```python
from build123d import *

# Parameters (mm, degrees)
FILLET1_R = 0.5


with BuildPart() as part:
    # Sketch1 → Revolve1 (revolve)
    with BuildSketch(Plane.XY):
        Polygon((24.25, 0), (31, 0), (31, 8), (26.75, 8), (26.75, 6), (29.25, 6), (29.25, 4), (26.5, 4), (26.5, 2), (24.25, 2), align=None)
    revolve(axis=Axis((0, 0, 0), (0, 1, 0)))

    # Fillet1
    fillet1_edges = [part.edges().sort_by_distance(p)[0] for p in [
        (-31, 8, 0),
        (-31, 0, 0),
    ]]
    fillet(fillet1_edges, radius=FILLET1_R)


solid = part.part
```
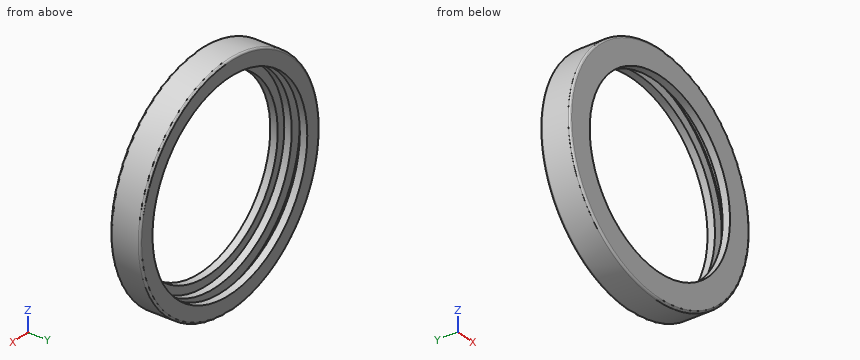
For this review, take the finished solid that the model builds, in its own axes (mm). Give positions to 0.01 mm unless a question says otherwise; leave off trailing zeros. Loops run counter-clockwise (first coordinate to the right, second up) from the corner with the lowest first, then second, coordinate; pieces in that order, holes last. Notation, with made-up numbers: M 10,10.25 L 61,10.25 A12 cw 61,28.25 Z; hole C 18,25.25 d4. An arc over 180 degrees is marked long. One line per item, written item: value. Start each with the question number.
Q1. Clearance check with flat-ended pins moving along their axes: pin 1 Ø1 at (y, z) = (1.5, 15) entering from -X; pin 2 Ø1.5 at (x, y) = (23, 2.5) entering from +Z; pin 3 Ø2 at (y, z) = (2, 15) entering from -X; pin 4 Ø5 at (x, z) = (-12, -17) entering from +Y. State where each tip first meets the part, or that it passes through.
Q2. Add section A-A (x = 0). Give the boundary of the cut face in (y, z).
Q3. Add section B-B (z = 0). Give the boundary of the cut face in (x, y), and give its area (3 significant figures).
Q4. For L1, parallel to Z at x = 0, y = 7.5; L2, parallel to Z at x = 0, y = 4.8, list the stretches that pass through material, from the lowest coordinate up.
Reply:
1. pin 1: x = -27.4
1. pin 2: z = 21.59
1. pin 3: x = -27.66
1. pin 4: through
2. outline: M 0,-30.5 A0.5 ccw 0.5,-31 L 7.5,-31 A0.5 ccw 8,-30.5 L 8,-26.75 L 6,-26.75 L 6,-29.25 L 4,-29.25 L 4,-26.5 L 2,-26.5 L 2,-24.25 L 0,-24.25 Z; M 0,24.25 L 2,24.25 L 2,26.5 L 4,26.5 L 4,29.25 L 6,29.25 L 6,26.75 L 8,26.75 L 8,30.5 A0.5 ccw 7.5,31 L 0.5,31 A0.5 ccw 0,30.5 Z
3. outline: M -31,0.5 A0.5 ccw -30.5,0 L -24.25,0 L -24.25,2 L -26.5,2 L -26.5,4 L -29.25,4 L -29.25,6 L -26.75,6 L -26.75,8 L -30.5,8 A0.5 ccw -31,7.5 Z; M 24.25,0 L 30.5,0 A0.5 ccw 31,0.5 L 31,7.5 A0.5 ccw 30.5,8 L 26.75,8 L 26.75,6 L 29.25,6 L 29.25,4 L 26.5,4 L 26.5,2 L 24.25,2 Z
3. area: 68.8 mm²
4. L1: -31 to -26.75, 26.75 to 31
4. L2: -31 to -29.25, 29.25 to 31
